from build123d import *

# Parameters (mm, degrees)
SKETCH_1_R               = 12.5
EXTRUDE_1_DEPTH          = 3
CUT_EXTRUDE_1_DEPTH      = 18.930421077
CUT_EXTRUDE_1_DEPTH_BACK = 18.930421077
SKETCH_2_R               = 5
SKETCH_3_R               = 1.6
CUT_EXTRUDE_2_DEPTH      = 19.668154703
PATTERN_CIRCULAR_1_COUNT = 2


with BuildPart() as part:
    # ｽｹｯﾁ1 → ﾎﾞｽ - 押し出し1 (new, symmetric)
    with BuildSketch(Plane.XY):
        Circle(SKETCH_1_R)
    extrude(amount=EXTRUDE_1_DEPTH, both=True)

    # ｽｹｯﾁ2 → ｶｯﾄ - 押し出し1 (cut, two sides: drawn at the far end of the back side and taken through both)
    with BuildSketch(Plane.XY.offset(-CUT_EXTRUDE_1_DEPTH_BACK)):
        Circle(SKETCH_2_R)
    extrude(amount=CUT_EXTRUDE_1_DEPTH + CUT_EXTRUDE_1_DEPTH_BACK, mode=Mode.SUBTRACT)

    # ｽｹｯﾁ3 → ｶｯﾄ - 押し出し2 (cut, symmetric)
    with BuildSketch(Plane.XY.offset(3)):
        with Locations((0, 8.5)):
            Circle(SKETCH_3_R)
    cut_extrude_2 = extrude(amount=CUT_EXTRUDE_2_DEPTH, both=True, mode=Mode.SUBTRACT)

    # 円形ﾊﾟﾀｰﾝ1: ｶｯﾄ - 押し出し2 ×2 about axis
    pattern_circular_1_axis = Axis((0, 0, 0), (0, 0, 1))
    for i in range(1, PATTERN_CIRCULAR_1_COUNT):
        add(cut_extrude_2.rotate(pattern_circular_1_axis, i * 360 / PATTERN_CIRCULAR_1_COUNT), mode=Mode.SUBTRACT)


solid = part.part
Build history of the part. All positions in model axes, mm. Round coordinates to 2 decimals unless told otherwise and drop trailing zeros. Write each loop counter-clockwise with the first axis right and the second up, starting at its lowest first coordinate (ties: lowest second). Pieces come first, ordered by that corner, then holes. Notation, with made-up numbers: M -9,80 L 28,80 A25 ccw 28,99 Z; hole C 78.25,-1 d3. An arc over 180 degrees is marked long. Answer in a Markdown table with one row per item.
1. Saw through at C-C (x = -3.75). List the corners of the cut face in (y, z).
Geometry check:
| item | result |
|---|---|
| outline | M -11.92,-3 L -3.31,-3 L -3.31,3 L -11.92,3 Z; M 3.31,-3 L 11.92,-3 L 11.92,3 L 3.31,3 Z |
2. Probe L1, parallel to Y at x = 0, z = -1.35; L2, parallel to Y at x = 1.25, z = -0.95; L3, parallel to X at y = -0.25, z = -2.15. List the from-to ranges inside material, lowest first. Write a range as [from, to].
Geometry check:
| item | result |
|---|---|
| L1 | [-12.5, -10.1], [-6.9, -5], [5, 6.9], [10.1, 12.5] |
| L2 | [-12.44, -9.5], [-7.5, -4.84], [4.84, 7.5], [9.5, 12.44] |
| L3 | [-12.5, -4.99], [4.99, 12.5] |
3. Saw through at D-D (x = 6.5). List the corners of the cut face in (y, z).
Geometry check:
| item | result |
|---|---|
| outline | M -10.68,-3 L 10.68,-3 L 10.68,3 L -10.68,3 Z |
4. Saw through at A-A (y = 0). List the corners of the cut face in (x, z), and give its area (3 significant figures).
Geometry check:
| item | result |
|---|---|
| outline | M -12.5,-3 L -5,-3 L -5,3 L -12.5,3 Z; M 5,-3 L 12.5,-3 L 12.5,3 L 5,3 Z |
| area | 90.0 mm2 |
5. Saw through at B-B (z = -1.55). List the corners of the cut face in (x, y), and give its area (3 significant figures).
Geometry check:
| item | result |
|---|---|
| outline | C 0,0 d25; hole C 0,0 d10; hole C 0,-8.5 d3.2; hole C 0,8.5 d3.2 |
| area | 396 mm2 |
6. Flat gauge pins, fed straight in: P1, Ø3, axis at y = -9, z = 0.5, coming from the -X side; P2, Ø6, axis at x = 0, y = 0, coming from the +Z side; P3, Ø1.5, axis at x = -7.5, z = -1, coming from the +Y side; P4, Ø1, axis at y = 8.5, z = -1, coming from the -X side. Where does each tip first touch, or does it go through?
Geometry check:
| item | result |
|---|---|
| P1 | x = -10 |
| P2 | through |
| P3 | y = 10.52 |
| P4 | x = -9.6 |
